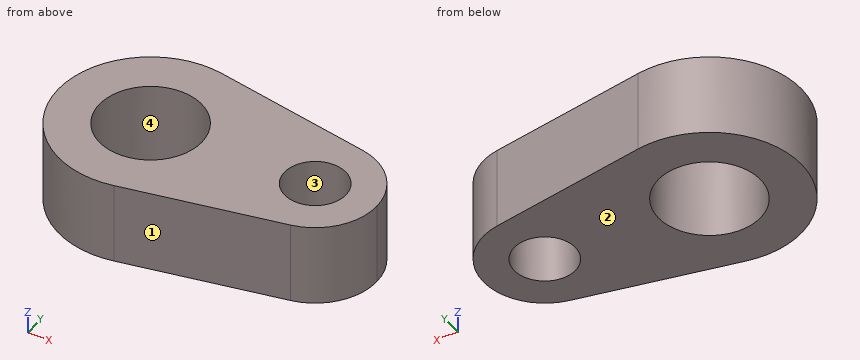
```python
from build123d import *

# Parameters (mm, degrees)
F0_R     = 15.875
F0_R_2   = 9.525
F1_DEPTH = 25.4


with BuildPart() as f1:
    # F0 (on Top) → F1 (new body)
    with BuildSketch(Plane.XY):
        with BuildLine():
            ThreePointArc((5.357813, -28.068211), (22.018516, -18.21306), (28.575, 0))
            ThreePointArc((28.575, 0), (22.018516, 18.21306), (5.357812, 28.068211))
            ThreePointArc((5.357812, 28.068211), (-28.575, 0), (5.357813, -28.068211))
        make_face()
        Circle(F0_R, mode=Mode.SUBTRACT)
        with BuildLine():
            ThreePointArc((69.85, 0), (65.479011, 12.14204), (54.371875, 18.712141))
            ThreePointArc((54.371875, 18.712141), (31.75, 0), (54.371875, -18.712141))
            ThreePointArc((54.371875, -18.712141), (65.479011, -12.14204), (69.85, 0))
        make_face()
        with Locations((50.8, 0)):
            Circle(F0_R_2, mode=Mode.SUBTRACT)
        with BuildLine():
            ThreePointArc((5.357812, 28.068211), (22.018516, 18.21306), (28.575, 0))
            ThreePointArc((28.575, 0), (22.018516, -18.21306), (5.357813, -28.068211))
            Line((5.357813, -28.068211), (54.371875, -18.712141))
            ThreePointArc((54.371875, -18.712141), (31.75, 0), (54.371875, 18.712141))
            Line((54.371875, 18.712141), (5.357812, 28.068211))
        make_face()
    extrude(amount=F1_DEPTH)


solid = f1.part
```
Source: CAD feature listing. Evaluate the final solid. Frame: model axes, mm. Face numbers are marked on the shaded views. Coordinates: 2 decimals unless noted, no trailing zeros. Loops run counter-clockwise (first coordinate to the right, second up) from the corner with the lowest first, then second, coordinate; pieces in that order, holes last. Notation, with made-up numbers: M 45,33 L 82,33 A20 cw 82,71 Z; hole C -32.75,41 d11. An arc over 180 degrees is marked long. Put each result on its own line as item: value. Start each with the question number.
1) Cut plane C-C on z = 20.5. Return the cut outline in (x, y) (3 decimals).
2) Contact query for flat-ended pins moving along their axis: pin 1 Ø12 at (y, z) = (-7.5, 10.5) entering from -X; pin 2 Ø1.5 at (y, z) = (18, 21.5) entering from +X; pin 3 Ø5 at (x, z) = (41, 19.5) entering from +Y. Output: stop coordinate, or through.
3) Pull-direction query (X, two-part tool) for the marked faces 1, 2, 3 and 4; classes: pulls with the +X half, pulls with the -X half, needs draft (parallel to the pull), parting line crosses it, or undercut.
4) Ray query, L1, parallel to Y at x = 0, z = 5.5 (3 decimals); L2, parallel to X at y = -3.5, z = 12.25; L3, parallel to X at y = 1, z = 23. Return the intervals inside material, ascending. Write a range as from..to.
5) Cut plane D-D on y = 13. Return the cut outline in (x, z), then the cut area to 3 significant figures.
6) Cut plane B-B on y = -7. Return the cut outline in (x, z).
7) Cut plane A-A on x = 0. Return the cut outline in (y, z) (3 decimals), then the cut area to 3 significant figures.
The answers:
1. outline: M 5.358,-28.068 L 54.372,-18.712 A19.05 ccw 54.372,18.712 L 5.358,28.068 A28.575 ccw long Z; hole C 0,0 d31.75; hole C 50.8,0 d19.05
2. pin 1: stops at x = -28.54
2. pin 2: stops at x = 58.88
2. pin 3: stops at y = 21.74
3. face 1: pulls with the +X half
3. face 2: needs draft
3. face 3: undercut
3. face 4: undercut
4. L1: y = -28.575..-15.875, 15.875..28.575
4. L2: x = -28.36..-15.48, 15.48..41.94, 59.66..69.53
4. L3: x = -28.56..-15.84, 15.84..41.33, 60.27..69.82
5. outline: M -25.45,0 L -9.11,0 L -9.11,25.4 L -25.45,25.4 Z; M 9.11,0 L 64.72,0 L 64.72,25.4 L 9.11,25.4 Z
5. area: 1,830 mm²
6. outline: M -27.7,0 L -14.25,0 L -14.25,25.4 L -27.7,25.4 Z; M 14.25,0 L 44.34,0 L 44.34,25.4 L 14.25,25.4 Z; M 57.26,0 L 68.52,0 L 68.52,25.4 L 57.26,25.4 Z
7. outline: M -28.575,0 L -15.875,0 L -15.875,25.4 L -28.575,25.4 Z; M 15.875,0 L 28.575,0 L 28.575,25.4 L 15.875,25.4 Z
7. area: 645 mm²
